For this review, take the finished solid that the model builds, in its own axes (mm). Face numbers are marked on the shaded views. Give positions to 0.01 mm unless a question says otherwise; leave off trailing zeros. Loops run counter-clockwise (first coordinate to the right, second up) from the corner with the lowest first, then second, coordinate; pieces in that order, holes last. Notation, with made-up numbers: M 42.5,4 L 71.5,4 A23 ccw 71.5,28 Z; hole C 39.5,81.25 d7. An arc over 180 degrees is marked long. Use CSV: the item, a comma, the result in double quotes. Start each with the question number.
1. Insertion check: P1, Ø8, axis at x = -19, y = -7.5, coming from the -Z side; P2, Ø2, axis at y = 14, z = 1, coming from the -X side; P3, Ø2.5, axis at x = 8, y = 0, coming from the +Z side; P4, Ø1.5, axis at x = 15, y = -16, coming from the +Z side. Each pin has a flat end and moves straight along its axis. Give the tip position at first contact, or say it passes through.
2. Take a section at B-B, the plane y = 0. State how many separate pieces and enclosed holes the cut face has, and give its area (3 significant figures).
3. The part is to be moulded in two halves that separate along X. For the marked faces 1 and 2, say which applies: pulls with the +X half, pulls with the -X half, needs draft (parallel to the pull), parting line crosses it, or undercut.
4. Take a section at C-C, the plane y = 6.5. Write out the cut boundary in (x, z), and give its area (3 significant figures).
5. Take a section at D-D, the plane x = 13.5. Write out the cut boundary in (y, z), and give its area (3 significant figures).
6. Take a section at A-A, the plane x = 0. Write out the cut boundary in (y, z), and give its area (3 significant figures).
7. To check wall thickness, follow line 1 (Y direction, x = 0, z = 1.7); line 2 (Y direction, x = 0, z = 2.35); line 3 (Z direction, x = -14.5, y = 18). State the ranges of each line that lie inside material, in increasing order. Write a range as [from, to].
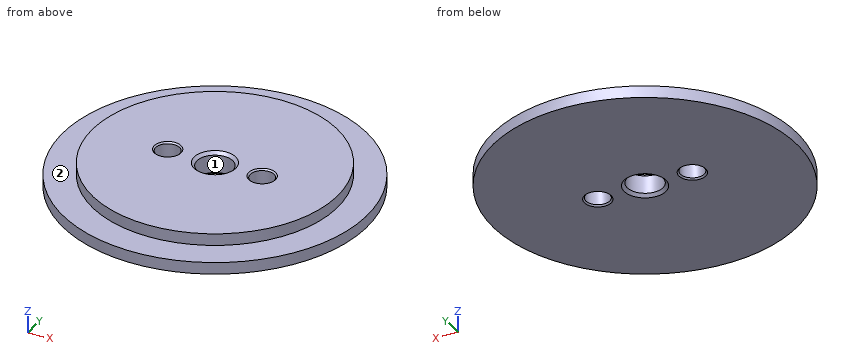
from build123d import *

# Parameters (mm, degrees)
SKETCH1_R           = 25.5
BOSS_EXTRUDE1_DEPTH = 2
SKETCH2_R           = 20.55
BOSS_EXTRUDE2_DEPTH = 2
SKETCH3_R           = 3
SKETCH3_R_2         = 2
CUT_EXTRUDE1_DEPTH  = 5
CHAMFER1_SIZE       = 0.25
CHAMFER2_SIZE       = 0.25
CHAMFER3_SIZE       = 0.5


with BuildPart() as part:
    # Sketch1 → Boss-Extrude1 (new body)
    with BuildSketch(Plane.XY):
        Circle(SKETCH1_R)
    extrude(amount=BOSS_EXTRUDE1_DEPTH)

    # Sketch2 → Boss-Extrude2 (add)
    with BuildSketch(Plane.XY.offset(2)):
        Circle(SKETCH2_R)
    extrude(amount=BOSS_EXTRUDE2_DEPTH)

    # Sketch3 → Cut-Extrude1 (cut, through all)
    with BuildSketch(Plane(origin=(0, 0, 0), x_dir=(-1, 0, 0), z_dir=(0, 0, -1))):
        Circle(SKETCH3_R)
        with Locations((8, 0)):
            Circle(SKETCH3_R_2)
        with Locations((-8, 0)):
            Circle(SKETCH3_R_2)
    extrude(amount=-CUT_EXTRUDE1_DEPTH, mode=Mode.SUBTRACT)

    # Chamfer1
    chamfer1_edges = [part.edges().sort_by_distance(p)[0] for p in [
        (10, 0, 4),
        (10, 0, 0),
    ]]
    chamfer(chamfer1_edges, length=CHAMFER1_SIZE)

    # Chamfer2
    chamfer2_edges = [part.edges().sort_by_distance(p)[0] for p in [
        (-6, 0, 4),
        (-6, 0, 0),
    ]]
    chamfer(chamfer2_edges, length=CHAMFER2_SIZE)

    # Chamfer3
    chamfer3_edges = [part.edges().sort_by_distance(p)[0] for p in [
        (3, 0, 4),
        (3, 0, 0),
    ]]
    chamfer(chamfer3_edges, length=CHAMFER3_SIZE)


solid = part.part
Result set:
1,P1,"z = 0"
1,P2,"x = -21.94"
1,P3,"through"
1,P4,"z = 2"
2,separate pieces,"4"
2,enclosed holes,"0"
2,area,"127 mm2"
3,face 1,"undercut"
3,face 2,"needs draft"
4,outline,"M -24.66,0 L 24.66,0 L 24.66,2 L 19.49,2 L 19.49,4 L -19.49,4 L -19.49,2 L -24.66,2 Z"
4,area,"177 mm2"
5,outline,"M -21.63,0 L 21.63,0 L 21.63,2 L 15.49,2 L 15.49,4 L -15.49,4 L -15.49,2 L -21.63,2 Z"
5,area,"149 mm2"
6,outline,"M -25.5,0 L -3.5,0 L -3,0.5 L -3,3.5 L -3.5,4 L -20.55,4 L -20.55,2 L -25.5,2 Z; M 3,0.5 L 3.5,0 L 25.5,0 L 25.5,2 L 20.55,2 L 20.55,4 L 3.5,4 L 3,3.5 Z"
6,area,"160 mm2"
7,line 1,"[-25.5, -3], [3, 25.5]"
7,line 2,"[-20.55, -3], [3, 20.55]"
7,line 3,"[0, 2]"
